from build123d import *

# Parameters (mm, degrees)
BOSS_EXTRUDE1_DEPTH = 9
FILLET2_R           = 2
FILLET3_R           = 2


with BuildPart() as part:
    # Sketch1 → Boss-Extrude1 (new body)
    with BuildSketch(Plane.XY):
        with BuildLine():
            ThreePointArc((-6.955420634, 8.36), (-9.215164105, 4.44856897), (-10, 0))
            Line((-10, 0), (10, 0))
            ThreePointArc((10, 0), (9.215164105, 4.44856897), (6.955420634, 8.36))
            Line((6.955420634, 8.36), (-6.955420634, 8.36))
        make_face()
        with BuildLine():
            Line((10, 0), (-10, 0))
            ThreePointArc((-10, 0), (-9.215164105, -4.44856897), (-6.955420634, -8.36))
            Line((-6.955420634, -8.36), (6.955420634, -8.36))
            ThreePointArc((6.955420634, -8.36), (9.215164105, -4.44856897), (10, 0))
        make_face()
    extrude(amount=BOSS_EXTRUDE1_DEPTH)

    # Fillet2
    fillet2_edges = [part.edges().sort_by_distance(p)[0] for p in [
        (-6.955420634, 8.36, 4.5),
        (6.955420634, 8.36, 4.5),
    ]]
    fillet(fillet2_edges, radius=FILLET2_R)

    # Fillet3
    fillet3_edges = [part.edges().sort_by_distance(p)[0] for p in [
        (6.955420634, -8.36, 4.5),
        (-6.955420634, -8.36, 4.5),
    ]]
    fillet(fillet3_edges, radius=FILLET3_R)


solid = part.part
Design review of the part built by this model. Coordinates are the model's own, in mm. Coordinates: 2 decimals unless noted, no trailing zeros. Order: outer loops, then holes, each group sorted by start corner. A loop starts at its lowest first (then second) coordinate and runs counter-clockwise, first axis right, second up.
Item 1: For pin 1 Ø1.5 at (y, z) = (5.5, 7) entering from +X, flat-tipped, find the tip position at first contact; note if it passes through.
Item 2: Take a section at B-B, the plane y = 3.75. Write out the cut boundary in (x, z).
Item 3: Take a section at C-C, the plane y = 6.5. Write out the cut boundary in (x, z), then the cut area to 3 significant figures.
Item 4: Take a section at A-A, the plane z = 6.5. Write out the cut boundary in (x, y), then the cut area to 3 significant figures.
Item 5: For line 1 (X direction, y = -0.25, z = 8.25); line 2 (X direction, y = 5, z = 5.75); line 3 (Y direction, x = -7, z = 3.5), list the stretches that pass through material, from the lowest coordinate up.
The answers:
1. pin 1: stops at x = 9.1
2. outline: (-9.45, 0) - (9.45, 0) - (9.45, 9) - (-9.45, 9) - close
3. outline: (-8.26, 0) - (8.26, 0) - (8.26, 9) - (-8.26, 9) - close
3. area: 149 mm2
4. outline: (-7.61, -7.52) arc R2 ccw to (-5.97, -8.36) - (5.97, -8.36) arc R2 ccw to (7.61, -7.52) arc R13 ccw to (7.61, 7.52) arc R2 ccw to (5.97, 8.36) - (-5.97, 8.36) arc R2 ccw to (-7.61, 7.52) arc R13 ccw to start
4. area: 302 mm2
5. line 1: x = -10 to 10
5. line 2: x = -9 to 9
5. line 3: y = -8.08 to 8.08
